The model under review builds one solid part; all positions refer to its coordinate system, in mm. A direction names the side the tool comes from. Round coordinates to 2 decimals unless told otherwise and drop trailing zeros. Order: outer loops, then holes, each group sorted by start corner. A loop starts at its lowest first (then second) coordinate and runs counter-clockwise, first axis right, second up. Notation, with made-up numbers: M 64,12.25 L 109,12.25 A14 cw 109,25.25 Z; hole C -27,5 d11. An arc over 180 degrees is marked long. Answer as a JSON object with one key per item and string values. Group by question number.
1. Add section B-B on x = -17.5. State the section outline as (y, z) points.
2. Clearance check with flat-ended pins moving along their axes: P1, Ø3, axis at x = -12, y = -6, coming from the -Z side; P2, Ø2, axis at x = -4, z = 33.5, coming from the -Y side; P3, Ø10, axis at x = -10, y = -2, coming from the -Z side; P4, Ø11.5, axis at x = -14, z = 11, coming from the +Y side. State where each tip first meets the part, or that it passes through.
3. Mouldability with a two-part tool opening along Y and no side actions: class faces 1 (the face through (-13, -24, 0)), 2 (the face through (-13, -25.4, 13)), 3 (the face through (-13, 0, 12)), 4 (the face through (-13, -13, 22.86)) as released by +Y, released by -Y, zero draft, split by the parting line, or undercut.
4. Machinability: for faces 5 (the face through (-13, -22.86, 11)), 6 (the face through (-13, -14, 25.4)), 7 (the face through (-12.522, 3.682, 38.816)), which of the approach directions +Z, -Z, +X, -X, +Y, -Y give a long, thin tool a straight path to every point of the face, cutting with its end or side? Answer none if there is none.
5. Add section A-A on z = 16.5. State the section outline as (x, y) points.
6. Add section D-D on z = 48. State the section outline as (x, y) points.
7. Add section C-C on y = -19. State the section outline as (x, z) points.
8. To check wall thickness, follow probe 1 along Y at (x, z) = (-2.5, 11); probe 2 along Z at (x, y) = (-15.5, -17.5); probe 3 along Z at (x, y) = (-11.5, -24). State the ranges of each line that lie inside material, in increasing order. Write a range as [from, to].
```python
from build123d import *

# Parameters (mm, degrees)
F0_W     = 25.4
F0_H     = 25.4
F1_DEPTH = 25.4
F2_T     = -2.54
F4_DEPTH = 25.4


with BuildPart() as f1:
    # F0 (on Top) → F1 (new body)
    with BuildSketch(Plane.XY):
        with Locations((-12.7, -12.7)):
            Rectangle(F0_W, F0_H)
    extrude(amount=F1_DEPTH)

    # F2
    f2_openings = [f1.faces().sort_by_distance(p)[0] for p in [
        (0, -12.7, 12.7),
        (-25.4, -12.7, 12.7),
        (-12.7, -12.7, 0),
    ]]
    offset(amount=F2_T, openings=f2_openings)

    # F3 (on Right) → F4 (join)
    with BuildSketch(Plane.YZ):
        Polygon((-3.526252, 24.17282), (0, 24.087025), (7.468844, 53.962406), (3.921144, 53.962406), align=None)
    extrude(amount=-F4_DEPTH)


solid = f1.part
```
Recorded:
{
 "1": {"outline": "M -25.4,0 L -22.86,0 L -22.86,22.86 L -2.54,22.86 L -2.54,0 L 0,0 L 0,24.09 L 7.47,53.96 L 3.92,53.96 L -3.22,25.4 L -25.4,25.4 Z"},
 "2": {"P1": "stops at z = 22.86", "P2": "stops at y = -1.44", "P3": "stops at z = 0", "P4": "stops at y = 0"},
 "3": {"face 1": "zero draft", "face 2": "released by -Y", "face 3": "released by +Y", "face 4": "undercut"},
 "4": {"face 5": "-Z, +X, -X", "face 6": "+Z, +X, -X, -Y", "face 7": "-Z, +X, -X, +Y"},
 "5": {"outline": "M -25.4,-25.4 L 0,-25.4 L 0,-22.86 L -25.4,-22.86 Z; M -25.4,-2.54 L 0,-2.54 L 0,0 L -25.4,0 Z"},
 "6": {"outline": "M -25.4,2.43 L 0,2.43 L 0,5.98 L -25.4,5.98 Z"},
 "7": {"outline": "M -25.4,22.86 L 0,22.86 L 0,25.4 L -25.4,25.4 Z"},
 "8": {"probe 1": "y = [-25.4, -22.86], [-2.54, 0]", "probe 2": "z = [22.86, 25.4]", "probe 3": "z = [0, 25.4]"}
}
